Source: CAD feature listing. Evaluate the final solid. Frame: model axes, mm. Face numbers are marked on the shaded views. Round coordinates to 2 decimals unless told otherwise and drop trailing zeros. Loops run counter-clockwise (first coordinate to the right, second up) from the corner with the lowest first, then second, coordinate; pieces in that order, holes last. Notation, with made-up numbers: (16, 37.5) -> (48, 37.5) arc R9 ccw to (48, 45.5) -> close; hole circle Ø10 at (13.5, -13.5). An arc over 180 degrees is marked (long way). Write item = value, one per line.
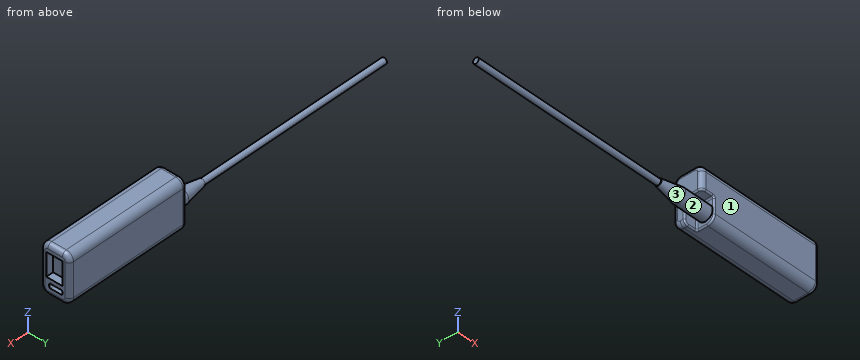
from build123d import *

# Parameters (mm, degrees)
SKETCH1_W           = 87
SKETCH1_H           = 33
BOSS_EXTRUDE1_DEPTH = 20
SKETCH3_W           = 16
SKETCH3_H           = 12
CUT_EXTRUDE1_DEPTH  = 9
SKETCH4_R           = 5
BOSS_EXTRUDE2_DEPTH = 35
SKETCH5_R           = 2
BOSS_EXTRUDE3_DEPTH = 135
SKETCH6_W           = 16
SKETCH6_H           = 11
CUT_EXTRUDE2_DEPTH  = 5
FILLET1_R           = 5
FILLET2_R           = 3
FILLET3_R           = 1
CHAMFER2_SIZE       = 15
CHAMFER2_SIZE2      = 2.644904711


with BuildPart() as part:
    # Sketch1 → Boss-Extrude1 (new body)
    with BuildSketch(Plane(origin=(0, 0, 0), x_dir=(1, 0, 0), z_dir=(0, 1, 0))):
        with Locations((43.5, 16.5)):
            Rectangle(SKETCH1_W, SKETCH1_H)
    extrude(amount=BOSS_EXTRUDE1_DEPTH)

    # Sketch3 → Cut-Extrude1 (cut)
    with BuildSketch(Plane.ZY):
        with Locations((-25, 6)):
            Rectangle(SKETCH3_W, SKETCH3_H)
    extrude(amount=-CUT_EXTRUDE1_DEPTH, mode=Mode.SUBTRACT)

    # Sketch4 → Boss-Extrude2 (add)
    with BuildSketch(Plane.ZY.offset(-9)):
        with Locations(Location((-25, 6, 0), (0, 0, 180))):
            Circle(SKETCH4_R)
    extrude(amount=BOSS_EXTRUDE2_DEPTH)

    # Sketch5 → Boss-Extrude3 (add)
    with BuildSketch(Plane.ZY.offset(26)):
        with Locations((-25, 6)):
            Circle(SKETCH5_R)
    extrude(amount=BOSS_EXTRUDE3_DEPTH)

    # Sketch6 → Cut-Extrude2 (cut)
    with BuildSketch(Plane(origin=(87, 0, 0), x_dir=(0, 0, -1), z_dir=(1, 0, 0))):
        with Locations((13.5, 9.5)):
            Rectangle(SKETCH6_W, SKETCH6_H)
        with BuildLine():
            Line((25.25, 15), (26.75, 15))
            ThreePointArc((26.75, 15), (27.280330086, 14.780330086), (27.5, 14.25))
            Line((27.5, 14.25), (27.5, 6.75))
            ThreePointArc((27.5, 6.75), (27.280330086, 6.219669914), (26.75, 6))
            Line((26.75, 6), (25.25, 6))
            ThreePointArc((25.25, 6), (24.719669914, 6.219669914), (24.5, 6.75))
            Line((24.5, 6.75), (24.5, 14.25))
            ThreePointArc((24.5, 14.25), (24.719669914, 14.780330086), (25.25, 15))
        make_face()
    extrude(amount=-CUT_EXTRUDE2_DEPTH, mode=Mode.SUBTRACT)

    # Fillet1
    fillet1_edges = [part.edges().sort_by_distance(p)[0] for p in [
        (43.5, 20, -33),
        (48, 0, -33),
        (43.5, 0, 0),
        (43.5, 20, 0),
    ]]
    fillet(fillet1_edges, radius=FILLET1_R)

    # Fillet2
    fillet2_edges = [part.edges().sort_by_distance(p)[0] for p in [
        (0, 0, -11),
        (0, 20, -16.5),
        (87, 20, -16.5),
        (0, 10, 0),
        (0, 13.5, -33),
        (0, 1.464466094, -1.464466094),
        (0, 18.535533906, -1.464466094),
        (0, 18.535533906, -31.535533906),
        (87, 10, -33),
        (87, 0, -16.5),
        (87, 10, 0),
        (87, 1.464466094, -31.535533906),
        (87, 1.464466094, -1.464466094),
        (87, 18.535533906, -1.464466094),
        (87, 18.535533906, -31.535533906),
    ]]
    fillet(fillet2_edges, radius=FILLET2_R)

    # Fillet3
    fillet3_edges = [part.edges().sort_by_distance(p)[0] for p in [
        (0, 7.5, -17),
        (0.878679656, 12, -32.121320344),
        (0.878679656, 0.878679656, -17),
        (9, 8.5, -33),
        (9, 12, -25),
        (6, 12, -33),
        (9, 6, -17),
        (6, 0, -17),
        (0, 12, -23.5),
        (9, 0, -22.5),
        (9, 1.464466094, -31.535533906),
    ]]
    fillet(fillet3_edges, radius=FILLET3_R - 0.0001)  # a hair under: the kernel refuses the full size

    # Chamfer2
    chamfer2_edges = [part.edges().sort_by_distance(p)[0] for p in [
        (-26, 6, -20),
    ]]
    chamfer2_side = [part.faces().sort_by_distance(p)[0] for p in [
        (-8.5, 6, -20),
    ]]
    chamfer(chamfer2_edges, length=CHAMFER2_SIZE, length2=CHAMFER2_SIZE2, reference=chamfer2_side[0])


solid = part.part
1. Section query C-C (x = -13.5). Return the cut outline in (y, z).
Evaluation:
outline = circle Ø9.12 at (6, -25)
2. Section query A-A (z = -13). Return the cut outline in (x, y), then the cut area to 3 significant figures.
Evaluation:
outline = (0, 3) arc R3 ccw to (3, 0) -> (84, 0) arc R3 ccw to (87, 3) -> (87, 4) -> (82, 4) -> (82, 15) -> (87, 15) -> (87, 17) arc R3 ccw to (84, 20) -> (3, 20) arc R3 ccw to (0, 17) -> close
area = 1,680 mm²
3. Section query B-B (x = -48). Return the cut outline in (y, z), then the cut area to 3 significant figures.
Evaluation:
outline = circle Ø4 at (6, -25)
area = 12.6 mm²
4. Mould query, pull axis Y, two halves, no side actions, for the marked faces 1, 2 and 3. Classes: released by +Y, released by -Y, zero draft, split by the parting line, or undercut.
Evaluation:
face_1 = released by -Y
face_2 = undercut
face_3 = split by the parting line
5. Contact query for flat-ended pins moving along their axis: pin 1 Ø3.5 at (x, y) = (3.5, 5) entering from -Z; pin 2 Ø4 at (y, z) = (10.5, -11) entering from -X; pin 3 Ø1.2 at (x, z) = (85.5, -26) entering from +Y; pin 4 Ø2.5 at (y, z) = (8.5, -26.5) entering from +X. Output: stop coordinate, or through.
Evaluation:
pin_1 = -30
pin_2 = 0
pin_3 = 19.86
pin_4 = 87
6. Line query: probe 1 along X at (y, z) = (4.5, -30); probe 2 along X at (y, z) = (7, -27); probe 3 along Y at (x, z) = (2.5, -28.5). Output: solid intervals per line, ascending. Write a range as from..to.
Evaluation:
probe_1 = 9..87
probe_2 = -26..82
probe_3 = 2.43..9.57, 12..19.93
